Check sheet for the modelled part. Datum: model origin and axes. Units: mm. A direction names the side the tool comes from. Give positions to 0.01 mm unless a question says otherwise; leave off trailing zeros. Loops run counter-clockwise (first coordinate to the right, second up) from the corner with the lowest first, then second, coordinate; pieces in that order, holes last. Notation, with made-up numbers: (56.5, 11.25) - (97.5, 11.25) arc R9 cw to (97.5, 27.25) - close; hole circle Ø11 at (88.5, -4.75). An arc over 180 degrees is marked (long way). Answer in a Markdown table with one row per item. Add a question column.
(1) Set-up check for faces 4 (the face through (-0.69, -3.1, 5.93)), 5 (the face through (-10.477, -0.075, 1.92)): record each of +Z, -Z, +X, -X, +Y, -Y from which the full face is reachable in a straight line by a thin tool's end or side.
(2) Sectioned sample at A-A on y = 0. Enter the section's corners in (x, z) (1 decimal).
(3) Go/stop test with flat-tipped pins: P1, Ø4.5, axis at x = 6.03, y = 0, coming from the -Z side; P2, Ø1.6, axis at x = -0.5, y = 0, coming from the +Z side; P3, Ø1.5, axis at x = 5, z = 7, coming from the +Y side; P4, Ø2, axis at x = 6.5, y = -1, coming from the -Z side. Record where each tip stops, or that it passes through.
(4) Sectioned sample at B-B on x = 0. Enter the section's corners in (y, z) (1 decimal), then the cut area to 3 significant figures.
(5) Thickness scan on L1, parallel to X at y = 0, z = 2.3; L2, parallel to Y at x = 0, z = 5.2 (1 decimal); L3, parallel to Z at x = 0.5, y = -0.75. Record the ranges inside material, lowest first.
(6) Draft check along X on faces 1 (the face through (-4.337, 0.534, 2.447)), 2 (the face through (0, 0, 0)), 3 (the face through (4.96, 5.17, 1.71)). Enter one of: released by +X, released by -X, zero draft, split by the parting line, or undercut.
from build123d import *

# Parameters (mm, degrees)
SKETCH3_R          = 1.778
EXTRUDE1_DEPTH     = 3.429
SKETCH4_R          = 3.175
SKETCH4_R_2        = 1.5875
EXTRUDE2_DEPTH     = 5.08
CUT_EXTRUDE2_DEPTH = 38.1


with BuildPart() as part:
    # Sketch3 → Extrude1 (new body)
    with BuildSketch(Plane.XY):
        with BuildLine():
            Line((2.363536842, 6.16656384), (7.623342105, 4.150571816))
            ThreePointArc((7.623342105, 4.150571816), (10.4775, 0), (7.623342105, -4.150571816))
            Line((7.623342105, -4.150571816), (2.363536842, -6.16656384))
            ThreePointArc((2.363536842, -6.16656384), (0, -6.604), (-2.363536842, -6.16656384))
            Line((-2.363536842, -6.16656384), (-7.623342105, -4.150571816))
            ThreePointArc((-7.623342105, -4.150571816), (-10.4775, 0), (-7.623342105, 4.150571816))
            Line((-7.623342105, 4.150571816), (-2.363536842, 6.16656384))
            ThreePointArc((-2.363536842, 6.16656384), (0, 6.604), (2.363536842, 6.16656384))
        make_face()
        with Locations((-6.0325, 0)):
            Circle(SKETCH3_R, mode=Mode.SUBTRACT)
        with Locations((6.0325, 0)):
            Circle(SKETCH3_R, mode=Mode.SUBTRACT)
    extrude(amount=EXTRUDE1_DEPTH)

    # Sketch4 → Extrude2 (add)
    with BuildSketch(Plane.XY.offset(3.429)):
        Circle(SKETCH4_R)
        Circle(SKETCH4_R_2, mode=Mode.SUBTRACT)
    extrude(amount=EXTRUDE2_DEPTH)

    # Cut-Extrude1 cone 1 section (through the dimple's axis) → Cut-Extrude1 (revolve, cut)
    with BuildSketch(Plane.YZ.offset(6.0325)):
        Polygon((0, 0), (3.556, 0), (0, 2.983838288), align=None)
    revolve(axis=Axis((6.0325, 0, 0), (0, 0, 1)), mode=Mode.SUBTRACT)

    # Cut-Extrude1 cone 2 section (through the dimple's axis) → Cut-Extrude1 cone 2 (revolve, cut)
    with BuildSketch(Plane.YZ.offset(-6.0325)):
        Polygon((0, 0), (3.556, 0), (0, 2.983838288), align=None)
    revolve(axis=Axis((-6.0325, 0, 0), (0, 0, 1)), mode=Mode.SUBTRACT)

    # Sketch6 → Cut-Extrude2 (cut, symmetric)
    with BuildSketch(Plane(origin=(0, 0, 0), x_dir=(1, 0, 0), z_dir=(0, 1, 0))):
        with BuildLine():
            Line((10.4775, -0.85725), (10.4775, 0.508))
            Line((10.4775, 0.508), (-10.4775, 0.508))
            Line((-10.4775, 0.508), (-10.4775, -0.85725))
            ThreePointArc((-10.4775, -0.85725), (0, 0), (10.4775, -0.85725))
        make_face()
    extrude(amount=CUT_EXTRUDE2_DEPTH, both=True, mode=Mode.SUBTRACT)


solid = part.part
Reply:
| question | item | result |
|---|---|---|
| 1 | face 4 | +Z |
| 1 | face 5 | +Z, -Z, -X |
| 2 | outline | (-10.5, 0.9) arc R64.5 ccw to (-8.9, 0.6) - (-7.8, 1.5) - (-7.8, 3.4) - (-10.5, 3.4) - close; (-4.3, 1.5) - (-2.5, 0) arc R64.5 ccw to (2.5, 0) - (4.3, 1.5) - (4.3, 3.4) - (3.2, 3.4) - (3.2, 8.5) - (1.6, 8.5) - (1.6, 3.4) - (-1.6, 3.4) - (-1.6, 8.5) - (-3.2, 8.5) - (-3.2, 3.4) - (-4.3, 3.4) - close; (7.8, 1.5) - (8.9, 0.6) arc R64.5 ccw to (10.5, 0.9) - (10.5, 3.4) - (7.8, 3.4) - close |
| 3 | P1 | z = 1.09 |
| 3 | P2 | z = 3.43 |
| 3 | P3 | through |
| 3 | P4 | z = 1.22 |
| 4 | outline | (-6.6, 0) - (6.6, 0) - (6.6, 3.4) - (3.2, 3.4) - (3.2, 8.5) - (1.6, 8.5) - (1.6, 3.4) - (-1.6, 3.4) - (-1.6, 8.5) - (-3.2, 8.5) - (-3.2, 3.4) - (-6.6, 3.4) - close |
| 4 | area | 61.4 mm^2 |
| 5 | L1 | -10.48 to -7.81, -4.25 to 4.25, 7.81 to 10.48 |
| 5 | L2 | -3.2 to -1.6, 1.6 to 3.2 |
| 5 | L3 | 0 to 3.43 |
| 6 | face 1 | undercut |
| 6 | face 2 | split by the parting line |
| 6 | face 3 | released by +X |
